Design review of the part shown in the three views and the two pictorial views. Dimensions are in mm from the part's minimum x, y and z. A direction names the side the tool comes from. Give positions to 0.01 mm unless a question says otherwise; leave off trailing zeros. Loops run counter-clockwise (first coordinate to the right, second up) from the corner with the lowest first, then second, coordinate; pieces in that order, holes last. Notation, with made-up numbers: (65.25, -10.5) - (114.25, -10.5) arc R15 cw to (114.25, 14.5) - close; hole circle Ø4 at (72.5, 38.25). An arc over 180 degrees is marked (long way). Return JSON: item names as keys, results as strings. Group by question number.
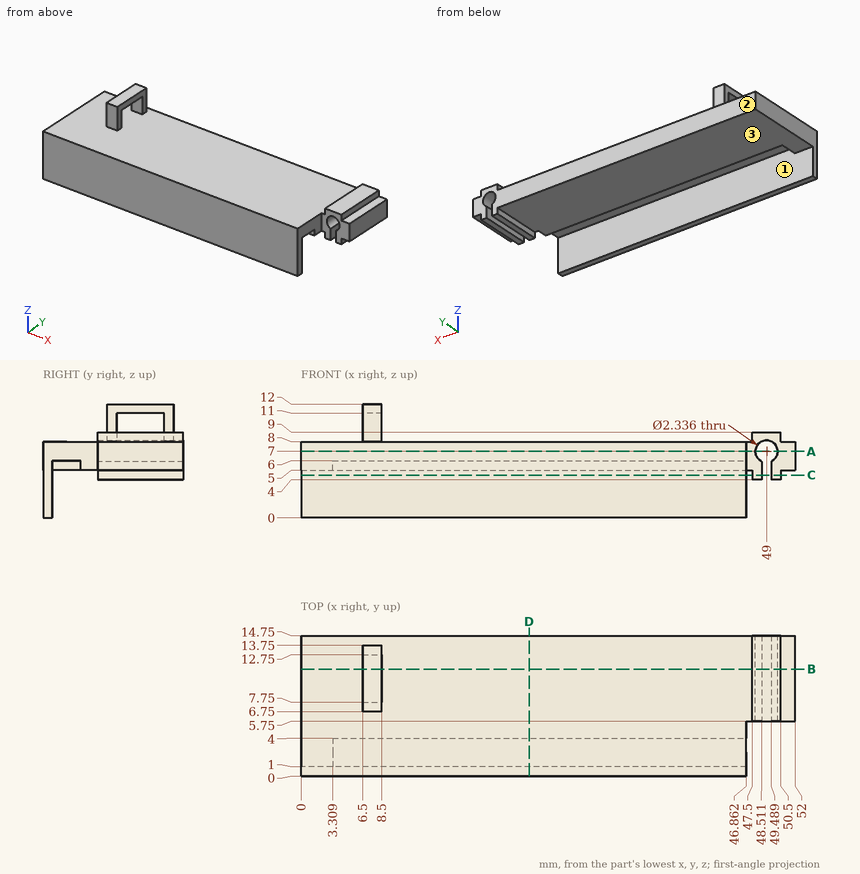
Item 1: For P1, Ø2.5, axis at x = 50.5, z = 7.5, coming from the -Y side; P2, Ø6, axis at x = 37.5, y = 3, coming from the +Z side; P3, Ø2, axis at y = 12, z = 9.5, coming from the -X side, all flat-tipped, find the tip position at first contact; note any pin that passes through.
Item 2: Tool access review of the marked faces 1, 2 and 3: name each direction out of +Z, -Z, +X, -X, +Y, -Y from which nothing blocks a thin tool from reaching the whole face with its end or side.
Item 3: Take a section at A-A (z = 7). State the section outline as (x, y) points.
Item 4: Take a section at C-C (z = 4.5). State the section outline as (x, y) points.
Item 5: For L1, parallel to Y at x = 44, z = 5.75; L2, parallel to X at y = 10.5, z = 7; L3, parallel to Z at x = 40, y = 2.75, list the stretches that pass through material, from the lowest coordinate up. Write a range as from..to.
Item 6: Take a section at D-D (x = 24). State the section outline as (y, z) points.
Item 7: Take a section at B-B (y = 11.25). State the section outline as (x, z) points, then the cut area to 3 significant figures.
Check sheet entries:
{
 "1": {"P1": "stops at y = 5.75", "P2": "stops at z = 8", "P3": "stops at x = 6.5"},
 "2": {"face 1": "-Z, +X", "face 2": "+Z, -Z, +X, -X, +Y", "face 3": "-Z, -X, +Y"},
 "3": {"outline": "(0, 0) - (46.86, 0) - (46.86, 5.75) - (47.83, 5.75) - (47.83, 14.75) - (0, 14.75) - close; (50.17, 5.75) - (52, 5.75) - (52, 14.75) - (50.17, 14.75) - close"},
 "4": {"outline": "(0, 0) - (46.86, 0) - (46.86, 1) - (0, 1) - close; (47.5, 5.75) - (48.51, 5.75) - (48.51, 14.75) - (47.5, 14.75) - close; (49.49, 5.75) - (50.5, 5.75) - (50.5, 14.75) - (49.49, 14.75) - close"},
 "5": {"L1": "y = 0..1, 4..14.75", "L2": "x = 0..47.83, 50.17..52", "L3": "z = 6..8"},
 "6": {"outline": "(0, 0) - (1, 0) - (1, 6) - (4, 6) - (4, 5) - (14.75, 5) - (14.75, 8) - (0, 8) - close"},
 "7": {"outline": "(0, 5) - (47.5, 5) - (47.5, 4) - (48.51, 4) - (48.51, 5.94) arc R1.17 cw (long way) to (49.49, 5.94) - (49.49, 4) - (50.5, 4) - (50.5, 5) - (52, 5) - (52, 8) - (50.5, 8) - (50.5, 9) - (47.5, 9) - (47.5, 8) - (0, 8) - close; (6.5, 11) - (8.5, 11) - (8.5, 12) - (6.5, 12) - close", "area": "158 mm^2"}
}
